Can you work these out from the model? Positions are in its coordinate system, mm. Face numbers are marked on the shaded views. A direction names the side the tool comes from. Give positions to 0.01 mm unless a question says otherwise; leave off trailing zeros. Order: outer loops, then holes, each group sorted by start corner. A loop starts at its lowest first (then second) coordinate and runs counter-clockwise, first axis right, second up. Notation, with made-up numbers: (-8, -9.75) - (9, -9.75) arc R20 cw to (9, 9.25) - close; hole circle Ø4 at (-9.75, 38.25). An arc over 180 degrees is marked (long way). Answer as a JSON object with one key per item and string values.
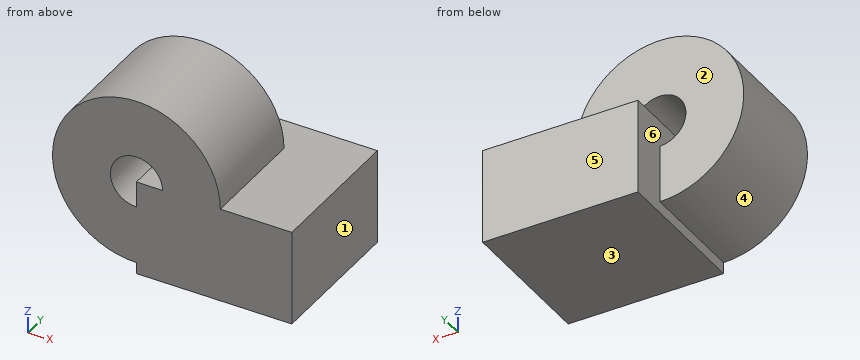
```python
from build123d import *

# Parameters (mm, degrees)
F0_W     = 41.426465
F0_H     = 39.133079
F1_DEPTH = 25.4
F2_W     = 15.425408
F2_H     = 29.133079


with BuildPart() as f1:
    # F0 (on Top) → F1 (new body)
    with BuildSketch(Plane.XY):
        with Locations((20.713233, 19.566539)):
            Rectangle(F0_W, F0_H)
    extrude(amount=F1_DEPTH)

    # F2 (on face) → F3 (revolve)
    with BuildSketch(Plane.XY.offset(25.4)):
        with Locations((14.647124, 14.566539)):
            Rectangle(F2_W, F2_H)
    revolve(axis=Axis((0, 19.56654, 25.4), (0, -1, 0)))


solid = f1.part
```
Q1. I'm going to push flat-ended pins straight in: pin 1 Ø1.5 at (y, z) = (14, 41.5) entering from -X; pin 2 Ø5 at (x, y) = (-5, 20) entering from -Z; pin 3 Ø12 at (x, z) = (-8, 9) entering from +Y. Where does each tip first touch, or does it pass through?
Recorded:
{"pin 1": "stops at x = -16.26", "pin 2": "stops at z = 3.18", "pin 3": "stops at y = 29.13"}
Q2. If we section it at D-D, the plane z = 14.5: Please give me the cut outline in (x, y), then the cut area to 3 significant figures.
Recorded:
{"outline": "(-19.52, 0) - (41.43, 0) - (41.43, 39.13) - (0, 39.13) - (0, 29.13) - (-19.52, 29.13) - close", "area": "2,190 mm^2"}
Q3. If we section it at B-B, the plane z = 29: Please give me the cut outline in (x, y), then the cut area to 3 significant figures.
Recorded:
{"outline": "(-22.07, 0) - (-5.93, 0) - (-5.93, 29.13) - (-22.07, 29.13) - close; (5.93, 0) - (22.07, 0) - (22.07, 29.13) - (5.93, 29.13) - close", "area": "940 mm^2"}
Q4. If we section it at C-C, the plane x = 18.5: Please give me the cut outline in (y, z), then the cut area to 3 significant figures.
Recorded:
{"outline": "(0, 0) - (39.13, 0) - (39.13, 25.4) - (29.13, 25.4) - (29.13, 37.96) - (0, 37.96) - close", "area": "1,360 mm^2"}
Q5. If we section it at A-A, the plane y = 7: Please give me the cut outline in (x, z), then the cut area to 3 significant figures.
Recorded:
{"outline": "(0, 0) - (41.43, 0) - (41.43, 25.4) - (22.36, 25.4) arc R22.36 ccw (long way) to (0, 3.04) - close; hole (0, 18.47) - (0, 25.4) - (6.93, 25.4) arc R6.93 ccw (long way) to start", "area": "2,120 mm^2"}
Q6. Which directions (+Z, -Z, +X, -X, +Y, -Y) give clear straight access to the entire face, cutting with the end or side of a thin tool? Please do the marked faces 1 and 2.
Recorded:
{"face 1": "+Z, -Z, +X, +Y, -Y", "face 2": "+Z, -X, +Y"}
Q7. We'd pull the mould along Z, two halves only. Please class the marked faces 3, 4, 5 and 6: released by +Z, released by -Z, zero draft, split by the parting line, or undercut.
Recorded:
{"face 3": "released by -Z", "face 4": "split by the parting line", "face 5": "zero draft", "face 6": "undercut"}
Q8. I need wall thicknesses on L1, parallel to X at y = 22, z = 25; L2, parallel to Y at x = -9.5, z = 44; L3, parallel to Z at x = 0.5, y = 18.5. Which ranges of each line are inside material? Lowest first, please.
Recorded:
{"L1": "x = -22.36 to -6.92, 0 to 41.43", "L2": "y = 0 to 29.13", "L3": "z = 0 to 25.4, 32.32 to 47.75"}
